Build history of the part. All positions in model axes, mm. A direction names the side the tool comes from. Coordinates: 2 decimals unless noted, no trailing zeros. Write each loop counter-clockwise with the first axis right and the second up, starting at its lowest first coordinate (ties: lowest second). Pieces come first, ordered by that corner, then holes. Notation, with made-up numbers: (-14.5, 89.5) -> (-0.5, 89.5) arc R17 cw to (-0.5, 110.5) -> close; hole circle Ø4 at (20, 32). An arc over 180 degrees is marked (long way). Write each question's results on one line, items separated by ' | '. Start each with the question number.
Q1. Tool access for faces 1 (the face through (3, 838.2, -26)), 2 (the face through (25, 413, -47.625)): list every direction of +Z, -Z, +X, -X, +Y, -Y with a clear straight run to the whole face (end or side of a thin tool).
Q2. Saw through at B-B on y = 497. Give the cut face in (x, z) (3 decimals).
Q3. Saw through at A-A on z = -36. Give the cut face in (x, y) (3 decimals), and give its area (3 significant figures).
Q4. Drill centre lines: line 1 (X direction, y = 497, z = -36.5) (3 decimals); line 2 (Z direction, x = 20.5, y = 104.5) (3 decimals). Where is each one in solid material? Low to high.
Q5. Two-plate mould, pull along X, no slides. Class faces 3 (the face through (3.175, 413, -25)), 4 (the face through (50.8, 413, -25)), 5 (the face through (25, 413, -50.8)): released by +X, released by -X, zero draft, split by the parting line, or undercut.
Q6. Drop a flat-ended pin along its axis: pin 1 Ø5.5 at (x, y) = (41.275, 9.525) entering from -Z. Give the stop position or say it passes through.
from build123d import *

# Parameters (mm, degrees)
SKETCH1_W           = 50.8
SKETCH1_H           = 50.8
SKETCH1_W_2         = 44.45
SKETCH1_H_2         = 44.45
BOSS_EXTRUDE1_DEPTH = 838.2
SKETCH2_R           = 3.175
SKETCH2_R_2         = 4.7625
CUT_EXTRUDE1_DEPTH  = 842.273154213


with BuildPart() as part:
    # Sketch1 → Boss-Extrude1 (new body)
    with BuildSketch(Plane(origin=(0, 0, 0), x_dir=(1, 0, 0), z_dir=(0, 1, 0))):
        with Locations((25.4, 25.4)):
            Rectangle(SKETCH1_W, SKETCH1_H)
        with Locations((25.4, 25.4)):
            Rectangle(SKETCH1_W_2, SKETCH1_H_2, mode=Mode.SUBTRACT)
    extrude(amount=BOSS_EXTRUDE1_DEPTH)

    # Sketch2 → Cut-Extrude1 (cut, through all)
    with BuildSketch(Plane.XY):
        with Locations((9.525, 111.125)):
            Circle(SKETCH2_R)
        with Locations((41.275, 111.125)):
            Circle(SKETCH2_R)
        with Locations((9.525, 9.525)):
            Circle(SKETCH2_R)
        with Locations((41.275, 9.525)):
            Circle(SKETCH2_R)
        with Locations((25.4, 23.114)):
            Circle(SKETCH2_R_2)
    extrude(amount=-CUT_EXTRUDE1_DEPTH, mode=Mode.SUBTRACT)


solid = part.part
Returned:
1) face 1: +Z, -Z, +X, -X, +Y | face 2: +Y, -Y
2) outline: (0, -50.8) -> (50.8, -50.8) -> (50.8, 0) -> (0, 0) -> close; hole (3.175, -47.625) -> (47.625, -47.625) -> (47.625, -3.175) -> (3.175, -3.175) -> close
3) outline: (0, 0) -> (3.175, 0) -> (3.175, 838.2) -> (0, 838.2) -> close; (47.625, 0) -> (50.8, 0) -> (50.8, 838.2) -> (47.625, 838.2) -> close | area: 5,320 mm2
4) line 1: x = 0 to 3.175, 47.625 to 50.8 | line 2: z = -50.8 to -47.625, -3.175 to 0
5) face 3: undercut | face 4: released by +X | face 5: zero draft
6) pin 1: passes through
